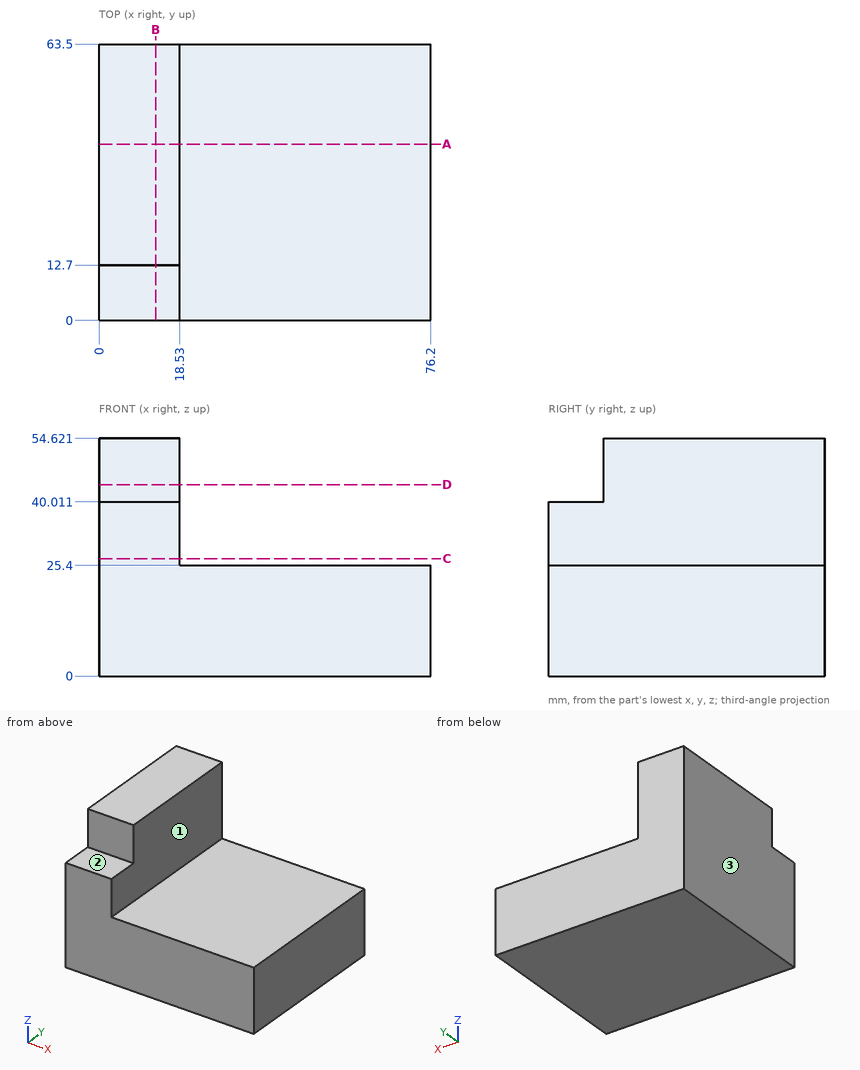
Check sheet for the drawn part. Datum: minimum x, y, z corner. Units: mm. A direction names the side the tool comes from. Coordinates: 2 decimals unless noted, no trailing zeros. Loops run counter-clockwise (first coordinate to the right, second up) from the corner with the lowest first, then second, coordinate; pieces in that order, holes last. Notation, with made-up numbers: (-1, -31.5) -> (12, -31.5) arc R21 cw to (12, 1.5) -> close; hole circle Ø5 at (30, 86). An arc over 180 degrees is marked (long way). Answer as a JSON object with one key per item and string values. Group by question number.
Item 1: Sectioned sample at B-B on x = 13. Record the boundary of the cut face in (y, z), plus the area to 3 significant figures.
Item 2: Depth check by flat-ended pin: pin 1 (2 mm diameter, centred on y = 39.5, z = 42, fed in from +X); pin 2 (4 mm diameter, centred on x = 11.5, y = 7, fed in from +Z); pin 3 (8 mm diameter, centred on x = 23, z = 46, fed in from +Y). Enter the tip coordinate at first touch or a pass-through.
Item 3: Tool access check on the marked faces 1, 2 and 3. Record the directions out of +Z, -Z, +X, -X, +Y, -Y that give a thin tool (end or side, any length) a straight path to the whole face; none if there is none.
Item 4: Sectioned sample at A-A on y = 40.5. Record the boundary of the cut face in (x, z), plus the area to 3 significant figures.
Item 5: Sectioned sample at C-C on z = 27. Record the boundary of the cut face in (x, y), plus the area to 3 significant figures.
Item 6: Scan lines: probe 1 along Z at (x, y) = (30.5, 35); probe 2 along Z at (x, y) = (8.5, 7); probe 3 along X at (y, z) = (55, 51). Record each from-to range of solid material in increasing order.
Item 7: Sectioned sample at D-D on z = 44. Record the boundary of the cut face in (x, y), plus the area to 3 significant figures.
Evaluation:
{
 "1": {"outline": "(0, 0) -> (63.5, 0) -> (63.5, 54.62) -> (12.7, 54.62) -> (12.7, 40.01) -> (0, 40.01) -> close", "area": "3,280 mm²"},
 "2": {"pin 1": "stops at x = 18.53", "pin 2": "stops at z = 40.01", "pin 3": "passes through"},
 "3": {"face 1": "+Z, +X, +Y, -Y", "face 2": "+Z, +X, -X, -Y", "face 3": "+Z, -Z, -X, +Y, -Y"},
 "4": {"outline": "(0, 0) -> (76.2, 0) -> (76.2, 25.4) -> (18.53, 25.4) -> (18.53, 54.62) -> (0, 54.62) -> close", "area": "2,480 mm²"},
 "5": {"outline": "(0, 0) -> (18.53, 0) -> (18.53, 63.5) -> (0, 63.5) -> close", "area": "1,180 mm²"},
 "6": {"probe 1": "z = 0 to 25.4", "probe 2": "z = 0 to 40.01", "probe 3": "x = 0 to 18.53"},
 "7": {"outline": "(0, 12.7) -> (18.53, 12.7) -> (18.53, 63.5) -> (0, 63.5) -> close", "area": "941 mm²"}
}
